from build123d import *

# Parameters (mm, degrees)
BASE_FLANGE2_DEPTH = 475
SKETCH6_W          = 250
SKETCH6_H          = 225
CUT_EXTRUDE2_DEPTH = 2.54
SKETCH13_R         = 2.25
CUT_EXTRUDE4_DEPTH = 619.939427238
SKETCH14_R         = 2.25
CUT_EXTRUDE5_DEPTH = 0.889
SKETCH15_W         = 70
SKETCH15_H         = 20
CUT_EXTRUDE6_DEPTH = 0.889


# Sheet-metal steps are written as plain solids
with BuildPart() as part:
    # Sketch1 → Base-Flange2 (new body)
    with BuildSketch(Plane(origin=(0, 0, 0), x_dir=(1, 0, 0), z_dir=(0, 1, 0))):
        with BuildLine():
            Line((195.849919958, 63.5), (195.849919958, 12.7))
            ThreePointArc((195.849919958, 12.7), (192.130176079, 3.719743879), (183.149919958, 0))
            Line((183.149919958, 0), (-183.149919958, 0))
            ThreePointArc((-183.149919958, 0), (-192.130176079, 3.719743879), (-195.849919958, 12.7))
            Line((-195.849919958, 12.7), (-195.849919958, 63.5))
            Line((-195.849919958, 63.5), (-194.960919958, 63.5))
            Line((-194.960919958, 63.5), (-194.960919958, 12.7))
            ThreePointArc((-194.960919958, 12.7), (-191.501558151, 4.348361807), (-183.149919958, 0.889))
            Line((-183.149919958, 0.889), (183.149919958, 0.889))
            ThreePointArc((183.149919958, 0.889), (191.501558151, 4.348361807), (194.960919958, 12.7))
            Line((194.960919958, 12.7), (194.960919958, 63.5))
            Line((194.960919958, 63.5), (195.849919958, 63.5))
        make_face()
    extrude(amount=BASE_FLANGE2_DEPTH)

    # Sketch6 → Cut-Extrude2 (cut)
    with BuildSketch(Plane.XY):
        with Locations((0, 162.5)):
            Rectangle(SKETCH6_W, SKETCH6_H)
    extrude(amount=-CUT_EXTRUDE2_DEPTH, mode=Mode.SUBTRACT)

    # Sketch13 → Cut-Extrude4 (cut, through all)
    with BuildSketch(Plane(origin=(195.849919958, 0, 0), x_dir=(0, 0, -1), z_dir=(1, 0, 0))):
        with Locations((50.096107, 60)):
            Circle(SKETCH13_R)
        with Locations((50.096107, 316.132840032)):
            Circle(SKETCH13_R)
        with Locations((50.096107, 30)):
            Circle(SKETCH13_R)
    extrude(amount=-CUT_EXTRUDE4_DEPTH, mode=Mode.SUBTRACT)

    # Sketch14 → Cut-Extrude5 (cut)
    with BuildSketch(Plane.XY):
        with Locations((-145.753813013, 316.132839976)):
            Circle(SKETCH14_R)
        with Locations((-118.946026903, 316.132839976)):
            Circle(SKETCH14_R)
        with Locations((118.946026903, 316.132839976)):
            Circle(SKETCH14_R)
        with Locations((145.753813013, 316.132839976)):
            Circle(SKETCH14_R)
        with Locations((145.753813013, 30)):
            Circle(SKETCH14_R)
        with Locations((118.946026903, 30)):
            Circle(SKETCH14_R)
        with Locations((-118.946026903, 30)):
            Circle(SKETCH14_R)
        with Locations((-145.753813013, 30)):
            Circle(SKETCH14_R)
    extrude(amount=-CUT_EXTRUDE5_DEPTH, mode=Mode.SUBTRACT)

    # Sketch15 → Cut-Extrude6 (cut)
    with BuildSketch(Plane.XY):
        with Locations((-50, 22)):
            Rectangle(SKETCH15_W, SKETCH15_H)
    extrude(amount=-CUT_EXTRUDE6_DEPTH, mode=Mode.SUBTRACT)


solid = part.part
Read the model definition and answer for the solid it produces. Units are mm, in the model's axes. A direction names the side the tool comes from. Round coordinates to 2 decimals unless told otherwise and drop trailing zeros. Order: outer loops, then holes, each group sorted by start corner. A loop starts at its lowest first (then second) coordinate and runs counter-clockwise, first axis right, second up.
1) The part is cut by section B-B on z = -34.5. Write down the section's boundary in (x, y), plus the area to 3 significant figures.
2) For faces 5 (the face through (-194.961, 234, -38)), 6 (the face through (-192.03, 234.18, -3.62)), determine the directions among +Z, -Z, +X, -X, +Y, -Y from which every point of the face is accessible in a straight line to the end or side of a thin tool.
3) Straight lines are drawn through the part: L1, parallel to X at y = 171, z = -30; L2, parallel to X at y = 74, z = -11; L3, parallel to Z at x = -92, y = 451. For each, find the intervals that lie inside material, in ascending order.
4) The part is cut by section A-A on y = 123.5. Write down the section's boundary in (x, z).
5) The part is cut by section C-C on x = 76.5. Write down the section's boundary in (y, z), plus the area to 3 significant figures.
6) The mould has two halves that part along X. Classify faces 1 (the face through (195.85, 234, -38)), 2 (the face through (3, 287, 0)), 3 (the face through (-191.59, 234.18, -4.44)), 4 (the face through (191.41, 234.18, -4.26)): released by +X, released by -X, zero draft, split by the parting line, or undercut.
7) The part is cut by section D-D on x = 162. Write down the section's boundary in (y, z), plus the area to 3 significant figures.
8) Flat-ended cylindrical pins translate along their axes: pin 1 (1 mm diameter, centred on y = 108, z = -0.5, fed in from +X); pin 2 (6 mm diameter, centred on x = 118.95, y = 316.13, fed in from -Z). Find the tip coordinate at first contact, or state that the pin passes through.
Resolved:
1. outline: (-195.85, 0) - (-194.96, 0) - (-194.96, 475) - (-195.85, 475) - close; (194.96, 0) - (195.85, 0) - (195.85, 475) - (194.96, 475) - close
1. area: 845 mm2
2. face 5: -Z, +Y, -Y
2. face 6: +Z, -X, +Y, -Y
3. L1: x = -195.85 to -194.96, 194.96 to 195.85
3. L2: x = -195.74 to -194.84, 194.84 to 195.74
3. L3: z = -0.89 to 0
4. outline: (-195.85, -63.5) - (-194.96, -63.5) - (-194.96, -12.7) arc R11.81 cw to (-183.15, -0.89) - (-125, -0.89) - (-125, 0) - (-183.15, 0) arc R12.7 ccw to (-195.85, -12.7) - close; (125, -0.89) - (183.15, -0.89) arc R11.81 cw to (194.96, -12.7) - (194.96, -63.5) - (195.85, -63.5) - (195.85, -12.7) arc R12.7 ccw to (183.15, 0) - (125, 0) - close
5. outline: (0, -0.89) - (50, -0.89) - (50, 0) - (0, 0) - close; (275, -0.89) - (475, -0.89) - (475, 0) - (275, 0) - close
5. area: 222 mm2
6. face 1: released by +X
6. face 2: zero draft
6. face 3: undercut
6. face 4: undercut
7. outline: (0, -0.89) - (475, -0.89) - (475, 0) - (0, 0) - close
7. area: 422 mm2
8. pin 1: stops at x = 188.09
8. pin 2: stops at z = -0.89
